Autodesk Inventor part; units mm, degrees
ref_plane "YZ Plane" through (0, 0, 0) normal (1, 0, 0) x (0, 1, 0)
ref_plane "XZ Plane" through (0, 0, 0) normal (0, 1, 0) x (-1, 0, 0)
ref_plane "XY Plane" through (0, 0, 0) normal (0, 0, 1) x (1, 0, 0)
sketch "Sketch1" plane through (0, 0, 0) normal (0, 1, 0) x (-1, 0, 0)
  line L0 (30, 30) -> (-30, 30)
  line L1 (-30, 30) -> (-30, -30)
  line L2 (-30, -30) -> (30, -30)
  line L3 (30, -30) -> (30, 30)
  line L4 (30, 30) -> (-30, -30) construction
  line L5 (-30, 30) -> (30, -30) construction
  point P0 (0, 0)
  dimension "d0" = 60
  dimension "d1" = 60
extrude "Extrusion1" add sketch "Sketch1" along normal blind 22.5
sketch "Sketch2" plane through (0, 22.5, 0) normal (0, 1, 0) x (1, 0, 0)
  line L0 (-25, 27.5) -> (25, 27.5)
  line L1 (27.5, 25) -> (27.5, -25)
  line L2 (25, -27.5) -> (-25, -27.5)
  line L3 (-27.5, 27.5) -> (27.5, -27.5) construction
  line L4 (27.5, 27.5) -> (-27.5, -27.5) construction
  arc A0 (-27.5, -25) -> (-25, -27.5) centre (-25, -25) ccw
  arc A1 (-25, 27.5) -> (-27.5, 25) centre (-25, 25) ccw
  arc A2 (27.5, 25) -> (25, 27.5) centre (25, 25) ccw
  arc A3 (25, -27.5) -> (27.5, -25) centre (25, -25) ccw
  line L5 (-27.5, -10) -> (-14, -10)
  line L6 (-11.5, -7.5) -> (-11.5, 7.5)
  line L7 (-14, 10) -> (-27.5, 10)
  line L8 (-27.5, -10) -> (-11.5, 10) construction
  line L9 (-11.5, -10) -> (-27.5, 10) construction
  line L10 (30, -30) -> (30, 30)
  arc A4 (-14, -10) -> (-11.5, -7.5) centre (-14, -7.5) ccw
  arc A5 (-11.5, 7.5) -> (-14, 10) centre (-14, 7.5) ccw
  line L11 (-27.5, -25) -> (-27.5, -10)
  line L12 (-27.5, 10) -> (-27.5, 25)
  point P0 (0, 0)
  point P1 (-19.5, 0)
  dimension "d4" = 55
  dimension "d5" = 55
  dimension "d6" = 2.5
  dimension "d19" = 16
  dimension "d20" = 20
  dimension "d21" = 41.5
  dimension "d22" = 2.5
extrude "Extrusion2" add sketch "Sketch2" along normal blind 7.5
sketch "Sketch3" plane through (0, 30, 0) normal (0, 1, 0) x (1, 0, 0)
  circle A0 centre (8.5, 0) radius 12.5
  line L0 (30, -30) -> (30, 30)
  point P0 (0, 0)
  dimension "d9" = 25
  dimension "d10" = 21.5
extrude "Extrusion3" cut sketch "Sketch3" against normal blind 10
sketch "Sketch4" plane through (0, 30, 0) normal (0, 1, 0) x (1, 0, 0)
  line L0 (-4, 17.5) -> (6, 17.5)
  line L1 (8.5, 15) -> (8.5, -15)
  line L2 (6, -17.5) -> (-4, -17.5)
  line L3 (-6.5, -15) -> (-6.5, 15)
  line L4 (-6.5, 17.5) -> (8.5, -17.5) construction
  line L5 (8.5, 17.5) -> (-6.5, -17.5) construction
  line L6 (30, -30) -> (30, 30)
  arc A0 (-6.5, -15) -> (-4, -17.5) centre (-4, -15) ccw
  arc A1 (-4, 17.5) -> (-6.5, 15) centre (-4, 15) ccw
  arc A2 (8.5, 15) -> (6, 17.5) centre (6, 15) ccw
  arc A3 (6, -17.5) -> (8.5, -15) centre (6, -15) ccw
  point P0 (0, 0)
  point P1 (1, 0)
  dimension "d13" = 15
  dimension "d14" = 35
  dimension "d15" = 36.5
  dimension "d16" = 2.5
extrude "Extrusion4" cut sketch "Sketch4" against normal blind 5
sketch "Sketch5" plane through (0, 22.5, 0) normal (0, 1, 0) x (1, 0, 0)
  circle A0 centre (-21.5, 0) radius 5
  line L0 (30, -30) -> (30, 30)
  point P0 (0, 0)
  dimension "d23" = 10
  dimension "d24" = 51.5
extrude "Extrusion5" add sketch "Sketch5" along normal blind 7.5
sketch "Sketch6" plane through (8.5, 20, 0) normal (0, 1, 0) x (1, 0, 0)
  circle A0 centre (0, 0) radius 2.5
  point P0 (-8.5, 0)
  dimension "d27" = 5
extrude "Extrusion6" cut sketch "Sketch6" against normal blind 12.5
sketch "Sketch7" plane through (0, 30, 0) normal (0, 1, 0) x (1, 0, 0)
  circle A0 centre (20, -22.5) radius 2.5
  line L0 (30, -30) -> (30, 30)
  line L1 (-30, -30) -> (30, -30)
  circle A1 centre (20, 22.5) radius 2.5
  circle A2 centre (-10, -22.5) radius 2.5
  circle A3 centre (-10, 22.5) radius 2.5
  circle A4 centre (-21.5, -22.5) radius 2.5
  circle A5 centre (-21.5, 22.5) radius 2.5
  point P0 (0, 0)
  dimension "d30" = 5
  dimension "d31" = 10
  dimension "d32" = 7.5
  dimension "d35" = 45
  dimension "d40" = 5
  dimension "d41" = 40
  dimension "d44" = 45
  dimension "d47" = 11.5
extrude "Extrusion7" cut sketch "Sketch7" against normal blind 10
properties part number "A2P1"
Design review of the part built by this model. Coordinates are the model's own, in mm. A direction names the side the tool comes from. Round coordinates to 2 decimals unless told otherwise and drop trailing zeros. Write each loop counter-clockwise with the first axis right and the second up, starting at its lowest first coordinate (ties: lowest second). Pieces come first, ordered by that corner, then holes. Notation, with made-up numbers: M 55.5,11 L 80.5,11 A13 cw 80.5,22 Z; hole C 4.25,-32.75 d11. An arc over 180 degrees is marked long. One line per item, written item: value. Start each with the question number.
1. Take a section at B-B on z = 22.5. State the section outline as (x, y) points.
2. Take a section at D-D on x = 7.5. State the section outline as (y, z) points.
3. Clearance check with flat-ended pins moving along their axes: P1, Ø2, axis at x = 11.5, y = 28, coming from the -Z side; P2, Ø5.5, axis at x = -9, z = -22, coming from the +Y side; P3, Ø2, axis at y = 26.5, z = -14, coming from the -X side; P4, Ø6, axis at x = -18, y = 26.5, coming from the +Z side. State where each tip first meets the part, or that it passes through.
4. Take a section at A-A on x = -8.5. State the section outline as (y, z) points.
5. For faces 4 (the face through (0, 26, 27.5)), 5 (the face through (18, 25, -24)), 6 (the face through (-26.787, 26.197, -26.748)), 7 (the face through (27.5, 26, 0)), list the 3-axis set-ups (+Z, -Z, +X, -X, +Y, -Y) from which the entire face can be reached by the end or side of a thin tool; tool diameter is ignored.
6. To check wall thickness, follow probe 1 along X at (y, z) = (26.25, -22.5); probe 2 along X at (y, z) = (25.5, 0); probe 3 along Z at (x, y) = (-21.5, 26.25). State the ranges of each line that lie inside material, in increasing order. Write a range as from..to.
7. Draft analysis for pull direction Z (two halves, no side actions). For faces 1 (the face through (0, 0, 0)), 2 (the face through (0, 11, -30)), 3 (the face through (8.5, 28, 14)), state which applies: pulls with the +Z half, pulls with the -Z half, needs draft (parallel to the pull), parting line crosses it, or undercut.
8. Take a section at C-C on z = 6. State the section outline as (x, y) points, then the cut area to 3 significant figures.
Computed:
1. outline: M -30,0 L 30,0 L 30,22.5 L 27.5,22.5 L 27.5,30 L 22.5,30 L 22.5,20 L 17.5,20 L 17.5,30 L -7.5,30 L -7.5,20 L -12.5,20 L -12.5,30 L -19,30 L -19,20 L -24,20 L -24,30 L -27.5,30 L -27.5,22.5 L -30,22.5 Z
2. outline: M 0,-30 L 22.5,-30 L 22.5,-27.5 L 30,-27.5 L 30,-17 L 25,-17 L 25,-12.46 L 20,-12.46 L 20,-2.29 L 7.5,-2.29 L 7.5,2.29 L 20,2.29 L 20,12.46 L 25,12.46 L 25,17 L 30,17 L 30,27.5 L 22.5,27.5 L 22.5,30 L 0,30 Z
3. P1: stops at z = -27.5
3. P2: stops at y = 30
3. P3: stops at x = -27.5
3. P4: stops at z = 27.5
4. outline: M 0,-30 L 22.5,-30 L 22.5,-27.5 L 30,-27.5 L 30,-24.5 L 20,-24.5 L 20,-20.5 L 30,-20.5 L 30,20.5 L 20,20.5 L 20,24.5 L 30,24.5 L 30,27.5 L 22.5,27.5 L 22.5,30 L 0,30 Z
5. face 4: +Z, +X, -X, +Y
5. face 5: +Y
5. face 6: -Z, -X, +Y
5. face 7: +Z, -Z, +X, +Y
6. probe 1: x = -27.5..-24, -19..-12.5, -7.5..17.5, 22.5..27.5
6. probe 2: x = -26.5..-16.5, -11.5..-6.5, 21..27.5
6. probe 3: z = -27.5..-25, -20..-10, -5..5, 10..20, 25..27.5
7. face 1: needs draft
7. face 2: pulls with the -Z half
7. face 3: undercut
8. outline: M -30,0 L 30,0 L 30,22.5 L 27.5,22.5 L 27.5,30 L 19.47,30 L 19.47,20 L -2.47,20 L -2.47,25 L -6.5,25 L -6.5,30 L -11.5,30 L -11.5,22.5 L -30,22.5 Z
8. area: 1,400 mm²
